Autodesk Inventor part; units mm, degrees
ref_plane "YZ Plane" through (0, 0, 0) normal (1, 0, 0) x (0, 1, 0)
ref_plane "XZ Plane" through (0, 0, 0) normal (0, 1, 0) x (-1, 0, 0)
ref_plane "XY Plane" through (0, 0, 0) normal (0, 0, 1) x (1, 0, 0)
sketch "Sketch1" plane through (0, 0, 0) normal (0, 0, 1) x (1, 0, 0)
  line L0 (-19.05, 19.05) -> (19.05, 19.05)
  line L1 (19.05, 19.05) -> (19.05, -19.05)
  line L2 (19.05, -19.05) -> (-19.05, -19.05)
  line L3 (-19.05, -19.05) -> (-19.05, 19.05)
  line L4 (0, 19.05) -> (0, -19.05) construction
  line L5 (-19.05, 0) -> (19.05, 0) construction
  point P0 (0, 0)
  point P1 (0, 0)
  dimension "d0" = 38.1
  dimension "d1" = 38.1
extrude "Extrusion1" add sketch "Sketch1" along normal blind 6.35
sketch "Sketch2" plane through (0, 0, 0) normal (0, 0, 1) x (1, 0, 0)
  point P0 (0, 0)
  point P1 (0, 0)
  point P2 (-12.7, 0)
  point P3 (12.7, 0)
  dimension "d4" = 12.7
  dimension "d5" = 12.7
hole "Hole1" at (0, 0, 0) at (-12.7, 0, 0) at (12.7, 0, 0) direction (0, 0, 1) diameter 6.35 end through all
fillet "Fillet1" radius 6.35 4 edges at (19.05, -19.05, 3.175) (19.05, 19.05, 3.175) (-19.05, 19.05, 3.175) (-19.05, -19.05, 3.175)
properties part number "J005646"
Part model, mm, in its own coordinate system. Coordinates: 2 decimals unless noted, no trailing zeros. Loops run counter-clockwise (first coordinate to the right, second up) from the corner with the lowest first, then second, coordinate; pieces in that order, holes last. Notation, with made-up numbers: (41.25, 55) - (49.25, 55) arc R13 ccw to (49.25, 70) - close; hole circle Ø3 at (-3.75, 8). An arc over 180 degrees is marked (long way). Write item = value, one per line. Start each with the question number.
Item 1: Cut at A-A, the plane x = 0. Give the cut face in (y, z) (3 decimals).
Item 2: Cut at D-D, the plane y = 15. Give the cut face in (x, z), and give its area (3 significant figures).
Item 3: Wall check: L1, parallel to X at y = 0, z = 2 (3 decimals); L2, parallel to Y at x = -12.7, z = 4.5 (3 decimals); L3, parallel to X at y = 2.5, z = 5. Give the ranges that are in metal, low to high. Write a range as from..to.
Item 4: Flat gauge pin, fed straight in: pin 1 Ø5 at (x, y) = (-12.7, 0) entering from -Z. Where does the tip first touch, or does it go through?
Item 5: Cut at C-C, the plane x = 12. Give the cut face in (y, z).
Item 6: Cut at B-B, the plane z = 3.25. Give the cut face in (x, y) (3 decimals).
Item 7: Mould opens along X. For faces 1 (the cylindrical face through (17.14, -17.24, 3.22)), 2 (the cylindrical face through (3.1, -0.69, 3.22)), 3 (the cylindrical face through (-17.24, -17.14, 3.22)) say: released by +X, released by -X, zero draft, split by the parting line, or undercut.
The answers:
q1.outline = (-19.05, 0) - (-3.175, 0) - (-3.175, 6.35) - (-19.05, 6.35) - close; (3.175, 0) - (19.05, 0) - (19.05, 6.35) - (3.175, 6.35) - close
q2.outline = (-18.62, 0) - (18.62, 0) - (18.62, 6.35) - (-18.62, 6.35) - close
q2.area = 236 mm2
q3.L1 = -19.05..-15.875, -9.525..-3.175, 3.175..9.525, 15.875..19.05
q3.L2 = -19.05..-3.175, 3.175..19.05
q3.L3 = -19.05..-14.66, -10.74..-1.96, 1.96..10.74, 14.66..19.05
q4.pin_1 = through
q5.outline = (-19.05, 0) - (-3.1, 0) - (-3.1, 6.35) - (-19.05, 6.35) - close; (3.1, 0) - (19.05, 0) - (19.05, 6.35) - (3.1, 6.35) - close
q6.outline = (-19.05, -12.7) arc R6.35 ccw to (-12.7, -19.05) - (12.7, -19.05) arc R6.35 ccw to (19.05, -12.7) - (19.05, 12.7) arc R6.35 ccw to (12.7, 19.05) - (-12.7, 19.05) arc R6.35 ccw to (-19.05, 12.7) - close; hole circle Ø6.35 at (-12.7, 0); hole circle Ø6.35 at (0, 0); hole circle Ø6.35 at (12.7, 0)
q7.face_1 = released by +X
q7.face_2 = undercut
q7.face_3 = released by -X
